from build123d import *

# Parameters (mm, degrees)
SKETCH1_W           = 220
SKETCH1_H           = 30
BOSS_EXTRUDE1_DEPTH = 3
SKETCH2_W           = 50
SKETCH2_H           = 220
BOSS_EXTRUDE2_DEPTH = 3
SKETCH3_R           = 2.5
CUT_EXTRUDE1_DEPTH  = 3
FILLET1_R           = 5
CUT_EXTRUDE2_REACH  = 5
SKETCH4_R           = 2
CUT_EXTRUDE3_REACH  = 8
SKETCH5_R           = 2


with BuildPart() as part:
    # Sketch1 → Boss-Extrude1 (new body)
    with BuildSketch(Plane(origin=(0, 0, 0), x_dir=(1, 0, 0), z_dir=(0, 1, 0))):
        Rectangle(SKETCH1_W, SKETCH1_H)
    extrude(amount=BOSS_EXTRUDE1_DEPTH)

    # Sketch2 → Boss-Extrude2 (add)
    with BuildSketch(Plane.XZ):
        with Locations((-85, 0)):
            Rectangle(SKETCH2_W, SKETCH2_H)
        with Locations((85, 0)):
            Rectangle(SKETCH2_W, SKETCH2_H)
    extrude(amount=BOSS_EXTRUDE2_DEPTH)

    # Sketch3 → Cut-Extrude1 (cut)
    with BuildSketch(Plane(origin=(0, 0, 0), x_dir=(1, 0, 0), z_dir=(0, 1, 0))):
        with Locations((-105, 105)):
            Circle(SKETCH3_R)
        with Locations((105, 105)):
            Circle(SKETCH3_R)
        with Locations((105, -105)):
            Circle(SKETCH3_R)
        with Locations((-105, -105)):
            Circle(SKETCH3_R)
    extrude(amount=-CUT_EXTRUDE1_DEPTH, mode=Mode.SUBTRACT)

    # Fillet1
    fillet1_edges = [part.edges().sort_by_distance(p)[0] for p in [
        (-60, -1.5, -110),
        (-60, -1.5, 110),
        (-110, -1.5, 110),
        (-110, -1.5, -110),
        (110, -1.5, -110),
        (110, -1.5, 110),
        (60, -1.5, 110),
        (60, -1.5, -110),
        (110, 1.5, 15),
        (-110, 1.5, 15),
        (-110, 1.5, -15),
        (110, 1.5, -15),
    ]]
    fillet(fillet1_edges, radius=FILLET1_R)

    # Sketch4 → Cut-Extrude2 (cut, up to next)
    with BuildSketch(Plane(origin=(0, 0, 0), x_dir=(1, 0, 0), z_dir=(0, 1, 0)), mode=Mode.PRIVATE) as cut_extrude2_sk1:
        with Locations((-97.5, 27.5)):
            Circle(SKETCH4_R)
    cut_extrude2_tool1 = extrude(cut_extrude2_sk1.sketch, amount=-CUT_EXTRUDE2_REACH, mode=Mode.PRIVATE) & part.part
    add(cut_extrude2_tool1.solids().sort_by_distance((-97.5, 0, -27.5))[0], mode=Mode.SUBTRACT)
    # Sketch4 → Cut-Extrude2 (cut, up to next)
    with BuildSketch(Plane(origin=(0, 0, 0), x_dir=(1, 0, 0), z_dir=(0, 1, 0)), mode=Mode.PRIVATE) as cut_extrude2_sk2:
        with Locations((-73.5, 27.5)):
            Circle(SKETCH4_R)
    cut_extrude2_tool2 = extrude(cut_extrude2_sk2.sketch, amount=-CUT_EXTRUDE2_REACH, mode=Mode.PRIVATE) & part.part
    add(cut_extrude2_tool2.solids().sort_by_distance((-73.5, 0, -27.5))[0], mode=Mode.SUBTRACT)
    # Sketch4 → Cut-Extrude2 (cut, up to next)
    with BuildSketch(Plane(origin=(0, 0, 0), x_dir=(1, 0, 0), z_dir=(0, 1, 0)), mode=Mode.PRIVATE) as cut_extrude2_sk3:
        with Locations((-73.5, 45.5)):
            Circle(SKETCH4_R)
    cut_extrude2_tool3 = extrude(cut_extrude2_sk3.sketch, amount=-CUT_EXTRUDE2_REACH, mode=Mode.PRIVATE) & part.part
    add(cut_extrude2_tool3.solids().sort_by_distance((-73.5, 0, -45.5))[0], mode=Mode.SUBTRACT)
    # Sketch4 → Cut-Extrude2 (cut, up to next)
    with BuildSketch(Plane(origin=(0, 0, 0), x_dir=(1, 0, 0), z_dir=(0, 1, 0)), mode=Mode.PRIVATE) as cut_extrude2_sk4:
        with Locations((-97.5, 45.5)):
            Circle(SKETCH4_R)
    cut_extrude2_tool4 = extrude(cut_extrude2_sk4.sketch, amount=-CUT_EXTRUDE2_REACH, mode=Mode.PRIVATE) & part.part
    add(cut_extrude2_tool4.solids().sort_by_distance((-97.5, 0, -45.5))[0], mode=Mode.SUBTRACT)
    # Sketch4 → Cut-Extrude2 (cut, up to next)
    with BuildSketch(Plane(origin=(0, 0, 0), x_dir=(1, 0, 0), z_dir=(0, 1, 0)), mode=Mode.PRIVATE) as cut_extrude2_sk5:
        with Locations((97.5, 45.5)):
            Circle(SKETCH4_R)
    cut_extrude2_tool5 = extrude(cut_extrude2_sk5.sketch, amount=-CUT_EXTRUDE2_REACH, mode=Mode.PRIVATE) & part.part
    add(cut_extrude2_tool5.solids().sort_by_distance((97.5, 0, -45.5))[0], mode=Mode.SUBTRACT)
    # Sketch4 → Cut-Extrude2 (cut, up to next)
    with BuildSketch(Plane(origin=(0, 0, 0), x_dir=(1, 0, 0), z_dir=(0, 1, 0)), mode=Mode.PRIVATE) as cut_extrude2_sk6:
        with Locations((73.5, 45.5)):
            Circle(SKETCH4_R)
    cut_extrude2_tool6 = extrude(cut_extrude2_sk6.sketch, amount=-CUT_EXTRUDE2_REACH, mode=Mode.PRIVATE) & part.part
    add(cut_extrude2_tool6.solids().sort_by_distance((73.5, 0, -45.5))[0], mode=Mode.SUBTRACT)
    # Sketch4 → Cut-Extrude2 (cut, up to next)
    with BuildSketch(Plane(origin=(0, 0, 0), x_dir=(1, 0, 0), z_dir=(0, 1, 0)), mode=Mode.PRIVATE) as cut_extrude2_sk7:
        with Locations((73.5, 27.5)):
            Circle(SKETCH4_R)
    cut_extrude2_tool7 = extrude(cut_extrude2_sk7.sketch, amount=-CUT_EXTRUDE2_REACH, mode=Mode.PRIVATE) & part.part
    add(cut_extrude2_tool7.solids().sort_by_distance((73.5, 0, -27.5))[0], mode=Mode.SUBTRACT)
    # Sketch4 → Cut-Extrude2 (cut, up to next)
    with BuildSketch(Plane(origin=(0, 0, 0), x_dir=(1, 0, 0), z_dir=(0, 1, 0)), mode=Mode.PRIVATE) as cut_extrude2_sk8:
        with Locations((97.5, 27.5)):
            Circle(SKETCH4_R)
    cut_extrude2_tool8 = extrude(cut_extrude2_sk8.sketch, amount=-CUT_EXTRUDE2_REACH, mode=Mode.PRIVATE) & part.part
    add(cut_extrude2_tool8.solids().sort_by_distance((97.5, 0, -27.5))[0], mode=Mode.SUBTRACT)
    # Sketch4 → Cut-Extrude2 (cut, up to next)
    with BuildSketch(Plane(origin=(0, 0, 0), x_dir=(1, 0, 0), z_dir=(0, 1, 0)), mode=Mode.PRIVATE) as cut_extrude2_sk9:
        with Locations((97.5, -27.5)):
            Circle(SKETCH4_R)
    cut_extrude2_tool9 = extrude(cut_extrude2_sk9.sketch, amount=-CUT_EXTRUDE2_REACH, mode=Mode.PRIVATE) & part.part
    add(cut_extrude2_tool9.solids().sort_by_distance((97.5, 0, 27.5))[0], mode=Mode.SUBTRACT)
    # Sketch4 → Cut-Extrude2 (cut, up to next)
    with BuildSketch(Plane(origin=(0, 0, 0), x_dir=(1, 0, 0), z_dir=(0, 1, 0)), mode=Mode.PRIVATE) as cut_extrude2_sk10:
        with Locations((73.5, -27.5)):
            Circle(SKETCH4_R)
    cut_extrude2_tool10 = extrude(cut_extrude2_sk10.sketch, amount=-CUT_EXTRUDE2_REACH, mode=Mode.PRIVATE) & part.part
    add(cut_extrude2_tool10.solids().sort_by_distance((73.5, 0, 27.5))[0], mode=Mode.SUBTRACT)
    # Sketch4 → Cut-Extrude2 (cut, up to next)
    with BuildSketch(Plane(origin=(0, 0, 0), x_dir=(1, 0, 0), z_dir=(0, 1, 0)), mode=Mode.PRIVATE) as cut_extrude2_sk11:
        with Locations((73.5, -45.5)):
            Circle(SKETCH4_R)
    cut_extrude2_tool11 = extrude(cut_extrude2_sk11.sketch, amount=-CUT_EXTRUDE2_REACH, mode=Mode.PRIVATE) & part.part
    add(cut_extrude2_tool11.solids().sort_by_distance((73.5, 0, 45.5))[0], mode=Mode.SUBTRACT)
    # Sketch4 → Cut-Extrude2 (cut, up to next)
    with BuildSketch(Plane(origin=(0, 0, 0), x_dir=(1, 0, 0), z_dir=(0, 1, 0)), mode=Mode.PRIVATE) as cut_extrude2_sk12:
        with Locations((97.5, -45.5)):
            Circle(SKETCH4_R)
    cut_extrude2_tool12 = extrude(cut_extrude2_sk12.sketch, amount=-CUT_EXTRUDE2_REACH, mode=Mode.PRIVATE) & part.part
    add(cut_extrude2_tool12.solids().sort_by_distance((97.5, 0, 45.5))[0], mode=Mode.SUBTRACT)
    # Sketch4 → Cut-Extrude2 (cut, up to next)
    with BuildSketch(Plane(origin=(0, 0, 0), x_dir=(1, 0, 0), z_dir=(0, 1, 0)), mode=Mode.PRIVATE) as cut_extrude2_sk13:
        with Locations((-97.5, -45.5)):
            Circle(SKETCH4_R)
    cut_extrude2_tool13 = extrude(cut_extrude2_sk13.sketch, amount=-CUT_EXTRUDE2_REACH, mode=Mode.PRIVATE) & part.part
    add(cut_extrude2_tool13.solids().sort_by_distance((-97.5, 0, 45.5))[0], mode=Mode.SUBTRACT)
    # Sketch4 → Cut-Extrude2 (cut, up to next)
    with BuildSketch(Plane(origin=(0, 0, 0), x_dir=(1, 0, 0), z_dir=(0, 1, 0)), mode=Mode.PRIVATE) as cut_extrude2_sk14:
        with Locations((-73.5, -45.5)):
            Circle(SKETCH4_R)
    cut_extrude2_tool14 = extrude(cut_extrude2_sk14.sketch, amount=-CUT_EXTRUDE2_REACH, mode=Mode.PRIVATE) & part.part
    add(cut_extrude2_tool14.solids().sort_by_distance((-73.5, 0, 45.5))[0], mode=Mode.SUBTRACT)
    # Sketch4 → Cut-Extrude2 (cut, up to next)
    with BuildSketch(Plane(origin=(0, 0, 0), x_dir=(1, 0, 0), z_dir=(0, 1, 0)), mode=Mode.PRIVATE) as cut_extrude2_sk15:
        with Locations((-73.5, -27.5)):
            Circle(SKETCH4_R)
    cut_extrude2_tool15 = extrude(cut_extrude2_sk15.sketch, amount=-CUT_EXTRUDE2_REACH, mode=Mode.PRIVATE) & part.part
    add(cut_extrude2_tool15.solids().sort_by_distance((-73.5, 0, 27.5))[0], mode=Mode.SUBTRACT)
    # Sketch4 → Cut-Extrude2 (cut, up to next)
    with BuildSketch(Plane(origin=(0, 0, 0), x_dir=(1, 0, 0), z_dir=(0, 1, 0)), mode=Mode.PRIVATE) as cut_extrude2_sk16:
        with Locations((-97.5, -27.5)):
            Circle(SKETCH4_R)
    cut_extrude2_tool16 = extrude(cut_extrude2_sk16.sketch, amount=-CUT_EXTRUDE2_REACH, mode=Mode.PRIVATE) & part.part
    add(cut_extrude2_tool16.solids().sort_by_distance((-97.5, 0, 27.5))[0], mode=Mode.SUBTRACT)

    # Sketch5 → Cut-Extrude3 (cut, up to next)
    with BuildSketch(Plane(origin=(0, 3, 0), x_dir=(1, 0, 0), z_dir=(0, 1, 0)), mode=Mode.PRIVATE) as cut_extrude3_sk1:
        with Locations((-6, 10)):
            Circle(SKETCH5_R)
    cut_extrude3_tool1 = extrude(cut_extrude3_sk1.sketch, amount=-CUT_EXTRUDE3_REACH, mode=Mode.PRIVATE) & part.part
    add(cut_extrude3_tool1.solids().sort_by_distance((-6, 3, -10))[0], mode=Mode.SUBTRACT)
    # Sketch5 → Cut-Extrude3 (cut, up to next)
    with BuildSketch(Plane(origin=(0, 3, 0), x_dir=(1, 0, 0), z_dir=(0, 1, 0)), mode=Mode.PRIVATE) as cut_extrude3_sk2:
        with Locations((6, 10)):
            Circle(SKETCH5_R)
    cut_extrude3_tool2 = extrude(cut_extrude3_sk2.sketch, amount=-CUT_EXTRUDE3_REACH, mode=Mode.PRIVATE) & part.part
    add(cut_extrude3_tool2.solids().sort_by_distance((6, 3, -10))[0], mode=Mode.SUBTRACT)
    # Sketch5 → Cut-Extrude3 (cut, up to next)
    with BuildSketch(Plane(origin=(0, 3, 0), x_dir=(1, 0, 0), z_dir=(0, 1, 0)), mode=Mode.PRIVATE) as cut_extrude3_sk3:
        with Locations((6, -10)):
            Circle(SKETCH5_R)
    cut_extrude3_tool3 = extrude(cut_extrude3_sk3.sketch, amount=-CUT_EXTRUDE3_REACH, mode=Mode.PRIVATE) & part.part
    add(cut_extrude3_tool3.solids().sort_by_distance((6, 3, 10))[0], mode=Mode.SUBTRACT)
    # Sketch5 → Cut-Extrude3 (cut, up to next)
    with BuildSketch(Plane(origin=(0, 3, 0), x_dir=(1, 0, 0), z_dir=(0, 1, 0)), mode=Mode.PRIVATE) as cut_extrude3_sk4:
        with Locations((-6, -10)):
            Circle(SKETCH5_R)
    cut_extrude3_tool4 = extrude(cut_extrude3_sk4.sketch, amount=-CUT_EXTRUDE3_REACH, mode=Mode.PRIVATE) & part.part
    add(cut_extrude3_tool4.solids().sort_by_distance((-6, 3, 10))[0], mode=Mode.SUBTRACT)


solid = part.part
Design review of the part built by this model. Coordinates are the model's own, in mm. A direction names the side the tool comes from. Coordinates: 2 decimals unless noted, no trailing zeros. Loops run counter-clockwise (first coordinate to the right, second up) from the corner with the lowest first, then second, coordinate; pieces in that order, holes last. Notation, with made-up numbers: M -1,32.25 L 31,32.25 A30 ccw 31,59.25 Z; hole C -16.75,40 d1. An arc over 180 degrees is marked long. Answer as CSV lines item,"result".
Item 1: Machinability: for faces 4 (the face through (-1, 0, 0)), 5 (the face through (-109, 2, -13)), 6 (the face through (108, 2, -14)), 7 (the face through (-62, -2, -109)), which of the approach directions +Z, -Z, +X, -X, +Y, -Y give a long, thin tool a straight path to every point of the face, cutting with its end or side? Answer none if there is none.
Answer list:
face 4,"+Z, -Z, -Y"
face 5,"-Z, -X, +Y"
face 6,"-Z, +X, +Y"
face 7,"-Z, +Y, -Y"
Item 2: The part is to be moulded in two halves that separate along Z. For faces 1 (the face through (-109, -2, -108)), 2 (the face through (-62, -2, 109)), 3 (the face through (-102.615, -1.479, 104.249)), say which applies: pulls with the +Z half, pulls with the -Z half, needs draft (parallel to the pull), parting line crosses it, or undercut.
Answer list:
face 1,"pulls with the -Z half"
face 2,"pulls with the +Z half"
face 3,"undercut"
Item 3: For P1, Ø6.5, axis at x = 97.5, z = 27.5, coming from the +Y side; P2, Ø1.5, axis at x = 25, y = 2, coming from the -Z side; P3, Ø1.5, axis at x = -57.5, y = 1.5, coming from the +Z side, all flat-tipped, find the tip position at first contact; note any pin that passes through.
Answer list:
P1,"y = 0"
P2,"z = -15"
P3,"z = 15"
Item 4: Add section B-B on x = 88. State the section outline as (y, z) points, plus the area to 3 significant figures.
Answer list:
outline,"M -3,-110 L 0,-110 L 0,-15 L 3,-15 L 3,15 L 0,15 L 0,110 L -3,110 Z"
area,"750 mm²"
Item 5: Add section A-A on z = 65. State the section outline as (x, y) points, plus the area to 3 significant figures.
Answer list:
outline,"M -110,-3 L -60,-3 L -60,0 L -110,0 Z; M 60,-3 L 110,-3 L 110,0 L 60,0 Z"
area,"300 mm²"
Item 6: For probe 1 along Z at (x, y) = (73.5, -1.1); probe 2 along X at (y, z) = (-1.65, -45.5); probe 3 along X at (y, z) = (-2.5, 50), list the stretches that pass through material, from the lowest coordinate up.
Answer list:
probe 1,"-110 to -47.5, -43.5 to -29.5, -25.5 to 25.5, 29.5 to 43.5, 47.5 to 110"
probe 2,"-110 to -99.5, -95.5 to -75.5, -71.5 to -60, 60 to 71.5, 75.5 to 95.5, 99.5 to 110"
probe 3,"-110 to -60, 60 to 110"
Item 7: Add section C-C on y = 1.25. State the section outline as (x, z) points, plus the area to 3 significant figures.
Answer list:
outline,"M -110,-10 A5 ccw -105,-15 L 105,-15 A5 ccw 110,-10 L 110,10 A5 ccw 105,15 L -105,15 A5 ccw -110,10 Z; hole C -6,-10 d4; hole C -6,10 d4; hole C 6,-10 d4; hole C 6,10 d4"
area,"6,530 mm²"
